```python
from build123d import *

# Parameters (mm, degrees)
CROQUIS1_R              = 3.75
CROQUIS1_R_2            = 3
SALIENTE_EXTRUIR1_DEPTH = 5
CROQUIS2_R              = 10.5
CROQUIS2_R_2            = 0.8
SALIENTE_EXTRUIR2_DEPTH = 2


with BuildPart() as part:
    # Croquis1 → Saliente-Extruir1 (new body)
    with BuildSketch(Plane(origin=(0, 0, 0), x_dir=(1, 0, 0), z_dir=(0, 1, 0))):
        Circle(CROQUIS1_R)
        Circle(CROQUIS1_R_2, mode=Mode.SUBTRACT)
    extrude(amount=SALIENTE_EXTRUIR1_DEPTH)

    # Croquis2 → Saliente-Extruir2 (add)
    with BuildSketch(Plane(origin=(0, 5, 0), x_dir=(1, 0, 0), z_dir=(0, 1, 0))):
        Circle(CROQUIS2_R)
        Circle(CROQUIS2_R_2, mode=Mode.SUBTRACT)
    extrude(amount=SALIENTE_EXTRUIR2_DEPTH)


solid = part.part
```
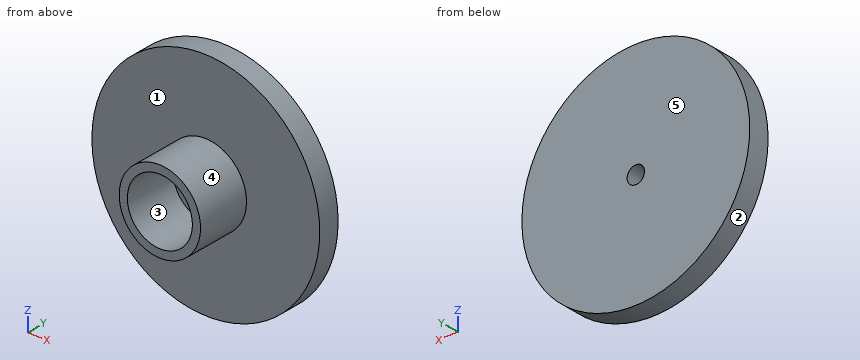
Check sheet for the modelled part. Datum: model origin and axes. Units: mm. Face numbers are marked on the shaded views. A direction names the side the tool comes from. Round coordinates to 2 decimals unless told otherwise and drop trailing zeros. Write each loop counter-clockwise with the first axis right and the second up, starting at its lowest first coordinate (ties: lowest second). Pieces come first, ordered by that corner, then holes. Notation, with made-up numbers: M -3.75,78 L 21.25,78 A22 ccw 21.25,87 Z; hole C 5,14.5 d6. An arc over 180 degrees is marked long. Write item = value, one per line. Start each with the question number.
1. Tool access check on the marked faces 4 and 5. Record the directions out of +Z, -Z, +X, -X, +Y, -Y that give a thin tool (end or side, any length) a straight path to the whole face; none if there is none.
2. Release check for a two-part mould opening along X. For the marked faces 1, 2 and 3 record: pulls with the +X half, pulls with the -X half, needs draft (parallel to the pull), parting line crosses it, or undercut.
3. Section check B-B, the plane z = 0. Record the cut outline in (x, y), then the cut area to 3 significant figures.
4. Section check D-D, the plane z = 2.5. Record the cut outline in (x, y).
5. Scan lines: line 1 (Z direction, x = 0, y = 5.8); line 2 (Y direction, x = -4, z = -3.25). Record each from-to range of solid material in increasing order. Write a range as [from, to].
6. Section check A-A, the plane x = 0. Record the cut outline in (y, z), then the cut area to 3 significant figures.
7. Section check C-C, the plane y = 5.25. Record the cut outline in (x, z), then the cut area to 3 significant figures.
8. Gauge pin test, flat ends, axial feed: pin 1 (1.5 mm diameter, centred on x = -5.5, y = 5, fed in from -Z); pin 2 (3 mm diameter, centred on x = -2, y = 3, fed in from +Z); pin 3 (3 mm diameter, centred on x = -1, z = 1, fed in from -Y). Record the tip position at first contact, or that the pin passes through.
Results found:
q1.face_4 = -Y
q1.face_5 = +Z, -Z, +X, -X, +Y
q2.face_1 = needs draft
q2.face_2 = parting line crosses it
q2.face_3 = undercut
q3.outline = M -10.5,5 L -3.75,5 L -3.75,0 L -3,0 L -3,5 L -0.8,5 L -0.8,7 L -10.5,7 Z; M 0.8,5 L 3,5 L 3,0 L 3.75,0 L 3.75,5 L 10.5,5 L 10.5,7 L 0.8,7 Z
q3.area = 46.3 mm^2
q4.outline = M -10.2,5 L -2.8,5 L -2.8,0 L -1.66,0 L -1.66,5 L 1.66,5 L 1.66,0 L 2.8,0 L 2.8,5 L 10.2,5 L 10.2,7 L -10.2,7 Z
q5.line_1 = [-10.5, -0.8], [0.8, 10.5]
q5.line_2 = [5, 7]
q6.outline = M 0,-3.75 L 5,-3.75 L 5,-10.5 L 7,-10.5 L 7,-0.8 L 5,-0.8 L 5,-3 L 0,-3 Z; M 0,3 L 5,3 L 5,0.8 L 7,0.8 L 7,10.5 L 5,10.5 L 5,3.75 L 0,3.75 Z
q6.area = 46.3 mm^2
q7.outline = C 0,0 d21; hole C 0,0 d1.6
q7.area = 344 mm^2
q8.pin_1 = -9.36
q8.pin_2 = 3.72
q8.pin_3 = 5
